The model under review builds one solid part; all positions refer to its coordinate system, in mm. A direction names the side the tool comes from. Give positions to 0.01 mm unless a question says otherwise; leave off trailing zeros. Order: outer loops, then holes, each group sorted by start corner. A loop starts at its lowest first (then second) coordinate and runs counter-clockwise, first axis right, second up. Notation, with made-up numbers: (85.5, 65.5) - (98.5, 65.5) arc R26 cw to (98.5, 89.5) - close; hole circle Ø8 at (-33.5, 39.25). An arc over 180 degrees is marked (long way). Answer as CSV lines item,"result". Start each with the question number.
Autodesk Inventor part; units mm, degrees
ref_plane "IN" through (-43.0479, -7.6232, 0) normal (-0.0872, 0.9962, 0) x (0, 0, 1)
ref_plane "OUT" through (-43.1176, -6.8262, 0) normal (-0.0872, 0.9962, 0) x (0, 0, 1)
ref_plane "YZ Plane" through (0, 0, 0) normal (1, 0, 0) x (0, 1, 0)
sketch "スケッチ2" plane through (0, 0, 0) normal (0, 0, 1) x (1, 0, 0)
  line L0 (-43.0479, 13.0453) -> (-43.0479, -8.9547)
  line L1 (-43.0479, -8.9547) -> (11.9521, -8.9547)
  line L2 (11.9521, -8.9547) -> (11.9521, 13.0453)
  line L3 (11.9521, 13.0453) -> (-43.0479, 13.0453)
  point P0 (0, 0)
  dimension "d3" = 55
  dimension "d16" = 22
extrude "押し出し2" add sketch "スケッチ2" along normal blind 12
sketch "スケッチ4" plane through (-43.0479, 13.0453, 0) normal (0, 1, 0) x (1, 0, 0)
  line L0 (55, 0) -> (55, -12)
  line L1 (0, 0) -> (0, -12)
  line L2 (0, -6) -> (55, -6)
  line L3 (0, -12) -> (55, -12)
  line L4 (0, 0) -> (55, 0)
  point P0 (10, -6)
  point P1 (45, -6)
  dimension "d17" = 10
  dimension "d18" = 35
hole "穴2" at (-33.0479, 13.0453, 6) at (1.9521, 13.0453, 6) direction (0, -1, 0) diameter 4.917 depth 12 tip angle 118
ref_plane "IN" through (-43.0479, -7.6232, 0) normal (-0.0872, 0.9962, 0) x (0, 0, 1)
ref_plane "OUT" through (-43.1176, -6.8262, 0) normal (-0.0872, 0.9962, 0) x (0, 0, 1)
sketch "スケッチ6" plane through (-43.1176, -6.8262, 0) normal (-0.0872, 0.9962, 0) x (0, 0, 1)
  line L0 (15.0202, 58.9603) -> (-3.3874, 58.9603)
  line L1 (-3.3874, 58.9603) -> (-3.3874, -4.1514)
  line L2 (-3.3874, -4.1514) -> (15.0202, -4.1514)
  line L3 (15.0202, -4.1514) -> (15.0202, 58.9603)
extrude "押し出し4" cut sketch "スケッチ6" against normal through all
chamfer "面取り1" distance 3 angle 45 1 edges at (11.9521, -2.0083, 6)
properties part number "100014" material "STEEL - HIGH GRADE ALLOY, BLACK OXIDE FINISH"
Item 1: Take a section at B-B on y = 3. Write out the cut boundary in (x, z).
Item 2: Take a section at C-C on x = -21.5. Write out the cut boundary in (y, z), and give its area (3 significant figures).
Item 3: Take a section at A-A on z = 2. Write out the cut boundary in (x, y).
Item 4: Machinability: for faces 5 (the face through (-43.048, 3, 6)), 6 (the face through (-35.485, 6.961, 5.68)), which of the approach directions +Z, -Z, +X, -X, +Y, -Y give a long, thin tool a straight path to every point of the face, cutting with its end or side? Answer none if there is none.
Item 5: Clearance check with flat-ended pins moving along their axes: pin 1 (4 mm diameter, centred on x = 1.95, z = 6, fed in from +Y); pin 2 (4 mm diameter, centred on x = -36, z = 3.5, fed in from -Y); pin 3 (3 mm diameter, centred on x = -33.05, z = 6, fed in from -Y). State where each tip first meets the part, or that it passes through.
Item 6: Mouldability with a two-part tool opening along X and no side actions: class faces 1 (the face through (-16.678, -4.513, 5.916)), 2 (the face through (1.54, -0.18, 5.91)), 3 (the face through (3.45, 6.96, 4.05)), 4 (the face through (-15, 13.045, 6)) as released by +X, released by -X, zero draft, split by the parting line, or undercut.
Item 7: For line 1 along X through (y, z) = (4, 6); line 2 along X through (y, z) = (7, 8.25); line 3 along Y through (x, z) = (-11, 7.75), list the stretches that pass through material, from the lowest coordinate up.
Item 8: Take a section at D-D on y = -4.25. Write out the cut boundary in (x, z), and give its area (3 significant figures).
Data:
1,outline,"(-43.05, 0) - (11.95, 0) - (11.95, 12) - (-43.05, 12) - close; hole circle Ø4.92 at (-33.05, 6); hole circle Ø4.92 at (1.95, 6)"
2,outline,"(-4.93, 0) - (13.05, 0) - (13.05, 12) - (-4.93, 12) - close"
2,area,"216 mm^2"
3,outline,"(-43.05, -6.82) - (8.96, -2.27) - (11.95, 0.99) - (11.95, 13.05) - (-43.05, 13.05) - close"
4,face 5,"+Z, -Z, -X, +Y, -Y"
4,face 6,"+Y"
5,pin 1,"stops at y = 0.77"
5,pin 2,"stops at y = -6.38"
5,pin 3,"stops at y = -6.08"
6,face 1,"released by +X"
6,face 2,"undercut"
6,face 3,"undercut"
6,face 4,"zero draft"
7,line 1,"x = -43.05 to -35.51, -30.59 to -0.51, 4.41 to 11.95"
7,line 2,"x = -43.05 to -34.04, -32.06 to 0.96, 2.94 to 11.95"
7,line 3,"y = -4.02 to 13.05"
8,outline,"(-43.05, 0) - (-13.67, 0) - (-13.67, 12) - (-43.05, 12) - close"
8,area,"353 mm^2"
